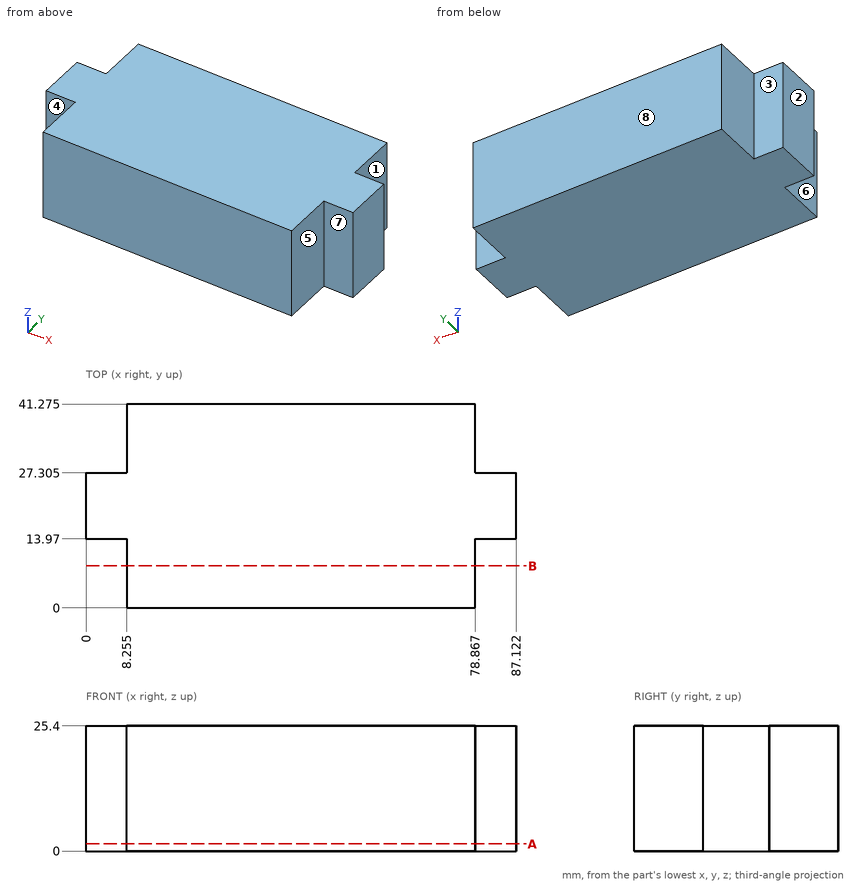
Source: three-view drawing plus pictorial views. Frame: mm from the lowest corner of the part. A direction names the side the tool comes from. Coordinates: 2 decimals unless noted, no trailing zeros. Order: outer loops, then holes, each group sorted by start corner. A loop starts at its lowest first (then second) coordinate and runs counter-clockwise, first axis right, second up.
1) Set-up query: the marked faces 1, 2, 3, 4 and 5. Return all of +Z, -Z, +X, -X, +Y, -Y with unobstructed straight access to the full face (end or side cutting, diameter ignored); none if empty.
Result sheet:
face 1: +Z, -Z, +X, +Y
face 2: +Z, -Z, -X, +Y, -Y
face 3: +Z, -Z, -X, +Y
face 4: +Z, -Z, -X, -Y
face 5: +Z, -Z, +X, -Y
2) Section B-B (y = 8.5). Return loops of the section in (x, z) (3 decimals), then the cut area to 3 significant figures.
Result sheet:
outline: (8.255, 0) - (78.867, 0) - (78.867, 25.4) - (8.255, 25.4) - close
area: 1,790 mm2
3) Section A-A (z = 1.5). Return loops of the section in (x, y) (3 decimals), then the cut area to 3 significant figures.
Result sheet:
outline: (0, 13.97) - (8.255, 13.97) - (8.255, 0) - (78.867, 0) - (78.867, 13.97) - (87.122, 13.97) - (87.122, 27.305) - (78.867, 27.305) - (78.867, 41.275) - (8.255, 41.275) - (8.255, 27.305) - (0, 27.305) - close
area: 3,130 mm2
4) Draft query along Y for the marked faces 6, 7 and 8. Return one class per face: released by +Y, released by -Y, zero draft, split by the parting line, or undercut.
Result sheet:
face 6: zero draft
face 7: released by -Y
face 8: released by +Y
5) First-contact query: P1, Ø3, axis at x = 30.5, y = 28, coming from the -Z side; P2, Ø8, axis at y = 8.5, z = 11, coming from the +X side; P3, Ø4, axis at x = 3.5, z = 7, coming from the -Y side; P4, Ø2.5, axis at x = 6, z = 11.5, coming from the +Y side (3 decimals). Flat tips, straight axial feed; report the tip coordinate or a pass-through.
Result sheet:
P1: stops at z = 0
P2: stops at x = 78.87
P3: stops at y = 13.97
P4: stops at y = 27.305
6) Ray query, probe 1 along X at (y, z) = (6.5, 21.5) (3 decimals); probe 2 along Y at (x, z) = (83.5, 15) (3 decimals). Return the intervals inside material, ascending.
Result sheet:
probe 1: x = 8.255 to 78.867
probe 2: y = 13.97 to 27.305
